Input: part model. Units: mm. Frame: model coordinates. A direction names the side the tool comes from. Coordinates: 2 decimals unless noted, no trailing zeros. Order: outer loops, then holes, each group sorted by start corner. A loop starts at its lowest first (then second) coordinate and runs counter-clockwise, first axis right, second up. Notation, with made-up numbers: (-30.5, 16) - (3.5, 16) arc R7 cw to (3.5, 28) - close; hole circle Ø6 at (-8.5, 57). An arc over 180 degrees is marked (long way). One line per question, with ' | ' between items. Start each with the question number.
```python
from build123d import *

# Parameters (mm, degrees)
BOSS_EXTRUDE1_DEPTH = 12.7
SKETCH3_R           = 1.904999998
CUT_EXTRUDE1_DEPTH  = 190.34


with BuildPart() as part:
    # Sketch1 → Boss-Extrude1 (new body)
    with BuildSketch(Plane(origin=(0, 21.945100429, 150.12727292), x_dir=(1, 0, 0), z_dir=(0, 0.144646288, 0.989483427))):
        Polygon((-64.482200742, -118.616237813), (29.337799258, -118.616237813), (29.337799258, -131.316237813), (80.137799258, -131.316237813), (80.137799258, -118.616237813), (168.877799258, -118.616237813), (168.877799258, -131.316237813), (219.677799258, -131.316237813), (219.677799258, -118.616237813), (313.497799258, -118.616237813), (313.497799258, 113.205700995), (-64.482200742, 113.205700995), align=None)
    extrude(amount=BOSS_EXTRUDE1_DEPTH)

    # Sketch3 → Cut-Extrude1 (cut)
    with BuildSketch(Plane.ZY.offset(-29.337799258)):
        with Locations((174.48639509, -100.788416836)):
            Circle(SKETCH3_R)
    extrude(amount=-CUT_EXTRUDE1_DEPTH, mode=Mode.SUBTRACT)


solid = part.part
```
(1) Material intervals for line 1 along X through (y, z) = (-95, 174); line 2 along Z through (x, y) = (234.5, -88.5); line 3 along Z through (x, y) = (81.5, 49.5), sorted ascending. Write a range as from..to.
(2) Reachability of faces 1 (the face through (-18.23, -94.52, 173.48)), 2 (the face through (123.89, -94.52, 173.48)), 3 (the face through (265.93, -94.52, 173.48)), 4 (the face through (127.154, 134.866, 139.948)) from +Z, -Z, +X, -X, +Y, -Y: full face, straight path, thin tool, end or side. Return the list, or none.
(3) Section A-A (x = 193). Output: boundary loops of the cut face in (y, z) (3 decimals).
(4) Section C-C (y = -61). Output: boundary loops of the cut face in (x, z), then the cut area to 3 significant figures.
(5) Section B-B (x = 16). Output: boundary loops of the cut face in (y, z).
(6) Draft query along X for faces 5 (the face through (-64.482, 22, 156)), 6 (the face through (54.382, -107.084, 175.317)), 7 (the face through (168.878, -99.5, 172.8)), 8 (the face through (313.498, 19, 157)). Return one class per face: +X half, -X half, draft (parallel to the pull), parting line (faces both ways), or undercut.
(7) Pin query (flat end, axial travel): pin 1 (5 mm diameter, centred on x = 130.5, y = 27, fed in from +Z); pin 2 (3 mm diameter, centred on x = 207, z = 173.5, fed in from -Y); pin 3 (4.5 mm diameter, centred on y = -102.5, z = 172, fed in from +X). Return the tip coordinate at first contact, or that it passes through.
Worked answers:
1) line 1: x = 29.34..80.14, 168.88..219.68 | line 2: z = 166.27..179.11 | line 3: z = 146.1..158.93
2) face 1: +Z, -X, -Y | face 2: +Z, -Y | face 3: +Z, +X, -Y | face 4: -Z, +X, -X, +Y
3) outline: (-107.99, 169.122) - (133.96, 133.752) - (135.797, 146.319) - (-106.153, 181.688) - close; hole circle Ø3.81 at (-100.788, 174.486)
4) outline: (-64.48, 162.25) - (313.5, 162.25) - (313.5, 175.09) - (-64.48, 175.09) - close | area: 4,850 mm²
5) outline: (-95.42, 167.28) - (133.96, 133.75) - (135.8, 146.32) - (-93.59, 179.85) - close
6) face 5: -X half | face 6: draft | face 7: undercut | face 8: +X half
7) pin 1: stops at z = 162.59 | pin 2: stops at y = -107.57 | pin 3: stops at x = 219.68
